Model file for the job. Use its own axes, mm. A direction names the side the tool comes from. Round coordinates to 2 decimals unless told otherwise and drop trailing zeros. Order: outer loops, then holes, each group sorted by start corner. A loop starts at its lowest first (then second) coordinate and runs counter-clockwise, first axis right, second up. Notation, with made-up numbers: (86, -13.5) - (142, -13.5) arc R6 ccw to (142, -7.5) - close; hole circle Ø9 at (37.25, -7.5). An arc over 180 degrees is marked (long way). Answer as CSV lines item,"result". Start each with the question number.
1. Wall check: line 1 along Z through (x, y) = (96, 28); line 2 along Y through (x, z) = (97.5, 3.15); line 3 along Y through (x, z) = (29, 14.5). Give the ranges that are in metal, low to high. Write a range as [from, to].
2. Pin check, flat tips, straight feed: pin 1 Ø3 at (y, z) = (28.5, 2.5) entering from +X; pin 2 Ø7.5 at (y, z) = (18, 8.5) entering from -X; pin 3 Ø2 at (x, z) = (74.5, 3.5) entering from -Y; pin 4 Ø4.5 at (x, z) = (41, 9) entering from +Y. Stop position of each tip, or through.
3. Pull direction X, two halves, no side cores. Call faces 1 (the face through (91.55, 28, 3)), 2 (the face through (25, 8.5, 3)), 3 (the face through (95.716, 29.908, 3.751)): released by +X, released by -X, zero draft, split by the parting line, or undercut.
4. Band-saw the part on A-A on x = 10. List the corners of the cut face in (y, z).
5. 3-axis set-ups, long thin cutter, end or side, ignore diameter. For faces 4 (the face through (95.7, 9.7, 1.2)), 5 (the face through (75, 8.5, 3)), 6 (the face through (49, 35, 13.75)): which of +Z, -Z, +X, -X, +Y, -Y reach the whole face in a straight line?
6. Band-saw the part on B-B on y = 38.5. List the corners of the cut face in (x, z).
```python
from build123d import *

# Parameters (mm, degrees)
F0_R      = 2
F1_DEPTH  = 100
F6_R      = 2
F6_R_2    = 1.8
F7_DEPTH  = 91.55
F8_DEPTH  = 6.5
F9_R      = 1
F10_R     = 1
F2_R      = 2.2
F13_R     = 2
F14_DEPTH = 8.5
F15_R     = 1.8
F16_DEPTH = 6.5
F17_R     = 1
F18_R     = 1


with BuildPart() as f1:
    # F0 (on Right) → F1 (new body)
    with BuildSketch(Plane.YZ):
        Polygon((37.5, 0), (40, 6.3), (40, 15.3), (33.9, 15.3), (33.9, 13.75), (35.8, 13.75), (35.8, 6.3), (0, 6.3), (0, 0), align=None)
        with Locations((10.15, 3.15)):
            Circle(F0_R, mode=Mode.SUBTRACT)
        with Locations((28, 3.15)):
            Circle(F0_R, mode=Mode.SUBTRACT)
    extrude(amount=F1_DEPTH)

    # F6 (on face) → F7 (join)
    with BuildSketch(Plane(origin=(0, 0, 0), x_dir=(0, -1, 0), z_dir=(-1, 0, 0))):
        with Locations((-28, 3.15)):
            Circle(F6_R)
        with Locations((-28, 3.15)):
            Circle(F6_R_2, mode=Mode.SUBTRACT)
        with Locations((-10.15, 3.15)):
            Circle(F6_R)
        with Locations((-10.15, 3.15)):
            Circle(F6_R_2, mode=Mode.SUBTRACT)
        with Locations((-28, 3.15)):
            Circle(F6_R_2)
        with Locations((-10.15, 3.15)):
            Circle(F6_R_2)
    extrude(amount=-F7_DEPTH)

    # F6 (on face) → F8 (join)
    with BuildSketch(Plane(origin=(0, 0, 0), x_dir=(0, -1, 0), z_dir=(-1, 0, 0))):
        with Locations((-28, 3.15)):
            Circle(F6_R_2)
        with Locations((-10.15, 3.15)):
            Circle(F6_R_2)
    extrude(amount=F8_DEPTH)

    # F9
    f9_edges = [f1.edges().sort_by_distance(p)[0] for p in [
        (-6.5, 29.8, 3.15),
    ]]
    fillet(f9_edges, radius=F9_R)

    # F10
    f10_edges = [f1.edges().sort_by_distance(p)[0] for p in [
        (-6.5, 11.95, 3.15),
    ]]
    fillet(f10_edges, radius=F10_R)

    # F11: sweep along a path in F5
    with BuildLine(Plane(origin=(0, 10.3674357858, -4.1140618198), x_dir=(-1, 0, 0), z_dir=(0, 0.9294907112, -0.3688455203))) as f11_path:
        Line((-74.083484861, 4.4261462437), (-74.083484861, -4.2147375643))
    # F2 (on face) → F11 (sweep, cut)
    with BuildSketch(Plane.XY.offset(6.3)):
        with Locations((25, 16.5)):
            Circle(F2_R)
    sweep(path=f11_path.line, mode=Mode.SUBTRACT)

    # F12: sweep along a path in F5
    with BuildLine(Plane(origin=(0, 10.3674357858, -4.1140618198), x_dir=(-1, 0, 0), z_dir=(0, 0.9294907112, -0.3688455203))) as f12_path:
        Line((-24.083484861, 11.2040515248), (-24.083484861, -2.310390817))
    # F2 (on face) → F12 (sweep, cut)
    with BuildSketch(Plane.XY.offset(6.3)):
        with Locations((75, 16.5)):
            Circle(F2_R)
    sweep(path=f12_path.line, mode=Mode.SUBTRACT)

    # F13 (on face) → F14 (cut)
    with BuildSketch(Plane.XZ):
        with Locations((25, 3.15)):
            Circle(F13_R)
        with Locations((75, 3.15)):
            Circle(F13_R)
    extrude(amount=-F14_DEPTH, mode=Mode.SUBTRACT)

    # F15 (on face) → F16 (join)
    with BuildSketch(Plane(origin=(0, 40, 0), x_dir=(-1, 0, 0), z_dir=(0, 1, 0))):
        with Locations((-75, 11.8)):
            Circle(F15_R)
        with Locations((-25, 11.8)):
            Circle(F15_R)
    extrude(amount=F16_DEPTH)

    # F17
    f17_edges = [f1.edges().sort_by_distance(p)[0] for p in [
        (76.8, 46.5, 11.8),
    ]]
    fillet(f17_edges, radius=F17_R)

    # F18
    f18_edges = [f1.edges().sort_by_distance(p)[0] for p in [
        (26.8, 46.5, 11.8),
    ]]
    fillet(f18_edges, radius=F18_R)


solid = f1.part
```
Reply:
1,line 1,"z = [0, 1.15], [5.15, 6.3]"
1,line 2,"y = [0, 8.15], [12.15, 26], [30, 38.75]"
1,line 3,"y = [33.9, 40]"
2,pin 1,"stops at x = 100"
2,pin 2,"stops at x = 0"
2,pin 3,"stops at y = 8.5"
2,pin 4,"stops at y = 40"
3,face 1,"released by +X"
3,face 2,"undercut"
3,face 3,"zero draft"
4,outline,"(0, 0) - (37.5, 0) - (40, 6.3) - (40, 15.3) - (33.9, 15.3) - (33.9, 13.75) - (35.8, 13.75) - (35.8, 6.3) - (0, 6.3) - close"
5,face 4,"+X"
5,face 5,"-Y"
5,face 6,"+X, -X, -Y"
6,outline,"(0, 2.52) - (100, 2.52) - (100, 15.3) - (0, 15.3) - close"
